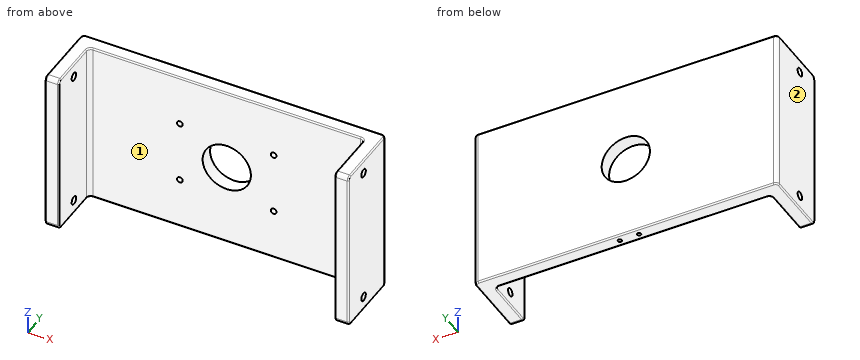
```python
from build123d import *

# Parameters (mm, degrees)
PAD_DEPTH       = 60
SKETCH001_R     = 3
POCKET_DEPTH    = 110.001
FILLET_R        = 3
FILLET001_R     = 1
SKETCH004_R     = 1.4
POCKET002_DEPTH = 3
SKETCH002_R     = 17.5
POCKET003_DEPTH = 10.001
SKETCH005_R     = 2.1
POCKET004_DEPTH = 6


with BuildPart() as part:
    # Sketch → Pad (new body, symmetric)
    with BuildSketch(Plane.XY):
        Polygon((0, 40), (-100, 40), (-100, 0), (-110, 0), (-110, 50), (0, 50), align=None)
        Polygon((0, 40), (0, 50), align=None)
    extrude(amount=PAD_DEPTH, both=True)

    # Sketch001 (on Face3 of Pad) → Pocket (cut, through all)
    with BuildSketch(Plane(origin=(-110, 0, 0), x_dir=(0, -1, 0), z_dir=(-1, 0, 0))):
        with Locations((-20, -50)):
            Circle(SKETCH001_R)
        with Locations((-20, 50)):
            Circle(SKETCH001_R)
    extrude(amount=-POCKET_DEPTH, mode=Mode.SUBTRACT)

    # Fillet
    fillet_edges = [part.edges().sort_by_distance(p)[0] for p in [
        (-105, 0, -60),
        (-100, 40, 0),
        (-105, 0, 60),
        (-110, 50, 0),
    ]]
    fillet(fillet_edges, radius=FILLET_R)

    # Fillet001
    fillet001_edges = [part.edges().sort_by_distance(p)[0] for p in [
        (-110, 25, 60),
        (-100, 0, 0),
    ]]
    fillet(fillet001_edges, radius=FILLET001_R)

    # Mirrored: part across YZ


with BuildPart() as part_1:
    add(part.part)
    add(part.part.mirror(Plane.YZ))

    # Sketch004 (on Face48 of Mirrored) → Pocket002 (cut)
    with BuildSketch(Plane(origin=(0, 0, -60), x_dir=(1, 0, 0), z_dir=(0, 0, -1))):
        with Locations((-7, -45)):
            Circle(SKETCH004_R)
        with Locations((7, -45)):
            Circle(SKETCH004_R)
    extrude(amount=-POCKET002_DEPTH, mode=Mode.SUBTRACT)

    # Sketch002 (on Face1 of Fillet001) → Pocket003 (cut, through all)
    with BuildSketch(Plane.XZ.offset(-40)):
        Circle(SKETCH002_R)
    extrude(amount=-POCKET003_DEPTH, mode=Mode.SUBTRACT)

    # Sketch005 (on Face34 of Pocket003) → Pocket004 (cut)
    with BuildSketch(Plane.XZ.offset(-40)):
        with Locations((-34, 22.65)):
            Circle(SKETCH005_R)
        with Locations((-34, -22.65)):
            Circle(SKETCH005_R)
        with Locations((34, -22.65)):
            Circle(SKETCH005_R)
        with Locations((34, 22.65)):
            Circle(SKETCH005_R)
    extrude(amount=-POCKET004_DEPTH, mode=Mode.SUBTRACT)


solid = part_1.part
```
Geometry check sheet. Reference: the model listing, model coordinates, mm. Face numbers are marked on the shaded views. A direction names the side the tool comes from. Coordinates: 2 decimals unless noted, no trailing zeros. Order: outer loops, then holes, each group sorted by start corner. A loop starts at its lowest first (then second) coordinate and runs counter-clockwise, first axis right, second up. Notation, with made-up numbers: M 28,47.5 L 71,47.5 A22 ccw 71,59.5 Z; hole C -24.75,-10 d11. An arc over 180 degrees is marked long. Answer as a JSON object with one key per item and string values.
Q1. Cross-section at D-D on z = 0. Record the cut outline in (x, y), and give its area (3 significant figures).
Results are:
{"outline": "M -110,1 A1 ccw -109,0 L -101,0 A1 ccw -100,1 L -100,37 A3 cw -97,40 L -17.5,40 L -17.5,50 L -107,50 A3 ccw -110,47 Z; M 17.5,40 L 97,40 A3 cw 100,37 L 100,1 A1 ccw 101,0 L 109,0 A1 ccw 110,1 L 110,47 A3 ccw 107,50 L 17.5,50 Z", "area": "2,650 mm²"}
Q2. Depth check by flat-ended pin: pin 1 Ø3.5 at (y, z) = (20, -50) entering from -X; pin 2 Ø2 at (x, z) = (34.5, -22) entering from -Y; pin 3 Ø5.5 at (x, z) = (-34, -22.65) entering from -Y. Enter the tip coordinate at first touch or a pass-through.
Results are:
{"pin 1": "passes through", "pin 2": "stops at y = 46", "pin 3": "stops at y = 40"}
Q3. Cross-section at A-A on y = 20. Give the number of separate pieces and of enclosed holes in the cut face, and give its area (3 significant figures).
Results are:
{"separate pieces": "6", "enclosed holes": "0", "area": "2,160 mm²"}
Q4. Cross-section at C-C on z = 22.65. Record the cut outline in (x, y).
Results are:
{"outline": "M -110,1 A1 ccw -109,0 L -101,0 A1 ccw -100,1 L -100,37 A3 cw -97,40 L -36.1,40 L -36.1,46 L -31.9,46 L -31.9,40 L 31.9,40 L 31.9,46 L 36.1,46 L 36.1,40 L 97,40 A3 cw 100,37 L 100,1 A1 ccw 101,0 L 109,0 A1 ccw 110,1 L 110,47 A3 ccw 107,50 L -107,50 A3 ccw -110,47 Z"}
Q5. Tool access check on the marked faces 1 and 2. Record the directions out of +Z, -Z, +X, -X, +Y, -Y that give a thin tool (end or side, any length) a straight path to the whole face; none if there is none.
Results are:
{"face 1": "+Z, -Z, -Y", "face 2": "+Z, -Z, -X, +Y, -Y"}
Q6. Cross-section at B-B on x = 0. Record the cut outline in (y, z).
Results are:
{"outline": "M 40,-59 A1 ccw 41,-60 L 49,-60 A1 ccw 50,-59 L 50,-17.5 L 40,-17.5 Z; M 40,17.5 L 50,17.5 L 50,59 A1 ccw 49,60 L 41,60 A1 ccw 40,59 Z"}
Q7. Scan lines: line 1 (X direction, y = 45, z = -59); line 2 (Z direction, x = 102, y = 20); line 3 (X direction, y = 26, z = -40.5). Record each from-to range of solid material in increasing order.
Results are:
{"line 1": "x = -110 to -8.4, -5.6 to 5.6, 8.4 to 110", "line 2": "z = -60 to -53, -47 to 47, 53 to 60", "line 3": "x = -110 to -100, 100 to 110"}
